Here's how the part is built. I have some questions about the finished solid (model axes, mm). Face numbers are marked on the shaded views. A direction names the side the tool comes from. Round coordinates to 2 decimals unless told otherwise and drop trailing zeros. Loops run counter-clockwise (first coordinate to the right, second up) from the corner with the lowest first, then second, coordinate; pieces in that order, holes last. Notation, with made-up numbers: (81, 36.5) - (105, 36.5) arc R26 ccw to (105, 71.5) - close; hole circle Ø8 at (39.25, 83). An arc over 180 degrees is marked (long way). Answer as a JSON object with one key per item and string values. Group by question number.
1) If we mould it in two halves opening along Y, with no side actions, what happens to the marked faces 3, 4 and 5? For each: pulls with the +Y half, pulls with the -Y half, needs draft (parallel to the pull), parting line crosses it, or undercut.
2) Which directions (+Z, -Z, +X, -X, +Y, -Y) give clear straight access to the entire face, cutting with the end or side of a thin tool? Please do the marked faces 1 and 2.
3) I want a section at C-C, the plane x = 77. Please give me the cut outline in (y, z), then the cut area to 3 significant figures.
4) If I drill on line 1 along Y through (x, z) = (49.5, 34); line 2 along X through (y, z) = (0, 55.75), over which ranges is the centre line in solid material (lowest first)? Write a range as [from, to].
5) I want a section at B-B, the plane y = 0. Please give me the cut outline in (x, z).
6) Will these pins go through, and if not, where does the flat tip stop? P1, Ø10, axis at x = 20, y = -46.5, coming from the +Z side; P2, Ø4, axis at x = -26.5, z = 45.5, coming from the +Y side.
7) I want a section at A-A, the plane z = -14. Please give me the cut outline in (x, y), then the cut area to 3 significant figures.
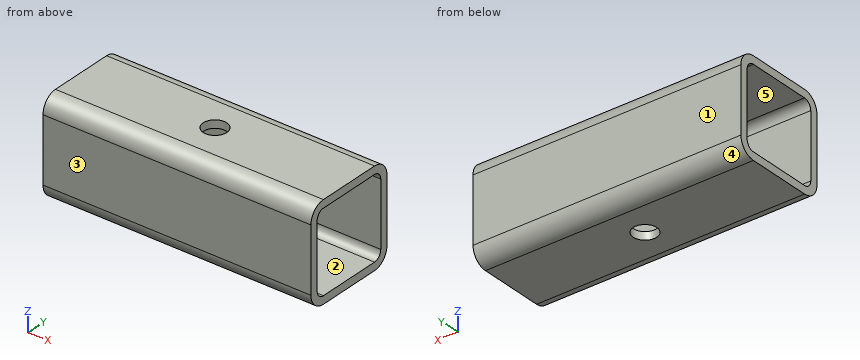
from build123d import *

# Parameters (mm, degrees)
F0_W          = 340
F0_H          = 122
F1_DEPTH      = 61
F2_R          = 20
F3_T          = -10
F4_R          = 15
F5_DEPTH      = 61.001
F5_DEPTH_BACK = 61.001


with BuildPart() as f1:
    # F0 (on Front) → F1 (new body, symmetric)
    with BuildSketch(Plane.XZ):
        Rectangle(F0_W, F0_H)
    extrude(amount=F1_DEPTH, both=True)

    # F2
    f2_edges = [f1.edges().sort_by_distance(p)[0] for p in [
        (0, 61, 61),
        (0, -61, 61),
        (0, 61, -61),
        (0, -61, -61),
    ]]
    fillet(f2_edges, radius=F2_R)

    # F3
    f3_openings = [f1.faces().sort_by_distance(p)[0] for p in [
        (170, 0, 0),
        (-170, 0, 0),
    ]]
    offset(amount=F3_T, openings=f3_openings)

    # F4 (on Top) → F5 (cut, two sides)
    with BuildSketch(Plane.XY) as f5_sk:
        Circle(F4_R)
    extrude(amount=F5_DEPTH, mode=Mode.SUBTRACT)
    extrude(f5_sk.sketch, amount=-F5_DEPTH_BACK, mode=Mode.SUBTRACT)


solid = f1.part
Outcome:
{
 "1": {"face 3": "pulls with the -Y half", "face 4": "pulls with the +Y half", "face 5": "undercut"},
 "2": {"face 1": "+Z, -Z, +X, -X, +Y", "face 2": "+X, -X"},
 "3": {"outline": "(-61, -41) arc R20 ccw to (-41, -61) - (41, -61) arc R20 ccw to (61, -41) - (61, 41) arc R20 ccw to (41, 61) - (-41, 61) arc R20 ccw to (-61, 41) - close; hole (-51, -41) arc R10 ccw to (-41, -51) - (41, -51) arc R10 ccw to (51, -41) - (51, 41) arc R10 ccw to (41, 51) - (-41, 51) arc R10 ccw to (-51, 41) - close", "area": "4,220 mm^2"},
 "4": {"line 1": "[-61, -51], [51, 61]", "line 2": "[-170, -15], [15, 170]"},
 "5": {"outline": "(-170, -61) - (-15, -61) - (-15, -51) - (-170, -51) - close; (-170, 51) - (-15, 51) - (-15, 61) - (-170, 61) - close; (15, -61) - (170, -61) - (170, -51) - (15, -51) - close; (15, 51) - (170, 51) - (170, 61) - (15, 61) - close"},
 "6": {"P1": "z = 60.99", "P2": "y = 60.84"},
 "7": {"outline": "(-170, -61) - (170, -61) - (170, -51) - (-170, -51) - close; (-170, 51) - (170, 51) - (170, 61) - (-170, 61) - close", "area": "6,800 mm^2"}
}
